For this review, take the finished solid that the model builds, in its own axes (mm). A direction names the side the tool comes from. Coordinates: 2 decimals unless noted, no trailing zeros. Write each loop counter-clockwise with the first axis right and the second up, starting at its lowest first coordinate (ties: lowest second). Pieces come first, ordered by that corner, then holes. Notation, with made-up numbers: (41, -18.5) -> (50, -18.5) arc R27 cw to (50, 8.5) -> close; hole circle Ø6 at (39, 35.25). An arc over 180 degrees is marked (long way). One line per item, written item: value. Start each with the question number.
1) Add section B-B (y = 5.25). State how many separate pieces and enclosed holes the cut face has, and give its area (3 significant figures).
2) Machinability: for faces 4 (the cylindrical face through (-64.03, 5.75, 0.64)), 5 (the cylindrical face through (8.88, 3.19, -21.78)), 6 (the cylindrical face through (-64.03, 0.6, 0.64)), which of the approach directions +Z, -Z, +X, -X, +Y, -Y give a long, thin tool a straight path to every point of the face, cutting with its end or side? Answer none if there is none.
3) Add section A-A (x = -43). State the section outline as (y, z) points, and give its area (3 significant figures).
4) For pin 1 Ø3 at (x, y) = (-89, 5.5) entering from -Z; pin 2 Ø2 at (y, z) = (4.5, 10) entering from -X; pin 3 Ø8 at (x, z) = (-45.5, -2.5) entering from -Y, all flat-tipped, find the tip position at first contact; note any pin that passes through.
5) Mouldability with a two-part tool opening along X and no side actions: class faces 1 (the cylindrical face through (8.88, 3.16, 21.78)), 2 (the cylindrical face through (-104.7, 3.13, 12.01)), 3 (the cylindrical face through (-50.09, 0.6, 24.76)) as released by +X, released by -X, zero draft, split by the parting line, or undercut.
6) For probe 1 along X at (y, z) = (3.75, 12.7) (3 decimals); probe 2 along X at (y, z) = (5.5, 12.5); probe 3 along X at (y, z) = (3.75, -12.7) (3 decimals), list the stretches that pass through material, from the lowest coordinate up. Write a range as from..to.
from build123d import *

# Parameters (mm, degrees)
SKETCH1_R           = 3.175
BOSS_EXTRUDE1_DEPTH = 6.35
FILLET2_R           = 12.7
FILLET3_R           = 2.116666667


with BuildPart() as part:
    # Sketch1 → Boss-Extrude1 (new body)
    with BuildSketch(Plane(origin=(0, 0, 0), x_dir=(1, 0, 0), z_dir=(0, 1, 0))):
        with BuildLine():
            Line((12.7, 25.4), (-12.7, 25.4))
            Line((-12.7, 25.4), (-12.7, 0))
            Line((-12.7, 0), (-114.3, 0))
            Line((-114.3, 0), (-114.3, -25.4))
            Line((-114.3, -25.4), (0, -25.4))
            ThreePointArc((0, -25.4), (8.980256121, -21.680256121), (12.7, -12.7))
            Line((12.7, -12.7), (12.7, 25.4))
        make_face()
        with Locations(Location((-76.2, -12.7, 0), (0, 0, 270))):
            Circle(SKETCH1_R, mode=Mode.SUBTRACT)
        with Locations(Location((-101.6, -12.7, 0), (0, 0, 270))):
            Circle(SKETCH1_R, mode=Mode.SUBTRACT)
        with Locations(Location((0, -12.7, 0), (0, 0, 270))):
            Circle(SKETCH1_R, mode=Mode.SUBTRACT)
        with Locations(Location((0, 12.7, 0), (0, 0, 270))):
            Circle(SKETCH1_R, mode=Mode.SUBTRACT)
    extrude(amount=BOSS_EXTRUDE1_DEPTH)

    # Fillet2
    fillet2_edges = [part.edges().sort_by_distance(p)[0] for p in [
        (12.7, 3.175, -25.4),
        (-12.7, 3.175, -25.4),
        (-114.3, 3.175, 0),
        (-114.3, 3.175, 25.4),
        (-12.7, 3.175, 0),
    ]]
    fillet(fillet2_edges, radius=FILLET2_R - 0.0001)  # a hair under: the kernel refuses the full size

    # Fillet3
    fillet3_edges = [part.edges().sort_by_distance(p)[0] for p in [
        (8.980256121, 6.35, 21.680256121),
        (12.7, 0, -5e-05),
        (12.7, 6.35, -5e-05),
        (8.980256121, 0, 21.680256121),
        (-63.5, 0, 0),
        (-63.5, 6.35, 0),
        (-50.80005, 0, 25.4),
        (-110.58028541, 0, 21.68028541),
        (-110.58028541, 0, 3.71971459),
        (-8.98028541, 0, -21.68028541),
        (8.98028541, 0, -21.68028541),
        (-50.80005, 6.35, 25.4),
        (-110.58028541, 6.35, 21.68028541),
        (-110.58028541, 6.35, 3.71971459),
        (-8.98028541, 6.35, -21.68028541),
        (8.98028541, 6.35, -21.68028541),
        (-16.41971459, 0, -3.71971459),
        (-16.41971459, 6.35, -3.71971459),
    ]]
    fillet(fillet3_edges, radius=FILLET3_R)


solid = part.part
Numbers:
1. separate pieces: 1
1. enclosed holes: 4
1. area: 3,520 mm²
2. face 4: -Z, -X, +Y
2. face 5: -Z, +X, +Y, -Y
2. face 6: -Z, -X, -Y
3. outline: (0, 2.12) arc R2.12 ccw to (2.12, 0) -> (4.23, 0) arc R2.12 ccw to (6.35, 2.12) -> (6.35, 23.28) arc R2.12 ccw to (4.23, 25.4) -> (2.12, 25.4) arc R2.12 ccw to (0, 23.28) -> close
3. area: 157 mm²
4. pin 1: z = 0
4. pin 2: x = -114.18
4. pin 3: y = 0.09
5. face 1: released by +X
5. face 2: undercut
5. face 3: zero draft
6. probe 1: -114.3..-104.775, -98.425..-79.375, -73.025..-3.175, 3.175..12.7
6. probe 2: -113.88..-104.77, -98.43..-79.37, -73.03..-3.17, 3.17..12.28
6. probe 3: -12.7..-3.175, 3.175..12.7
